Source: CAD feature listing. Evaluate the final solid. Frame: model axes, mm. Face numbers are marked on the shaded views. A direction names the side the tool comes from. Coordinates: 2 decimals unless noted, no trailing zeros. Write each loop counter-clockwise with the first axis right and the second up, starting at its lowest first coordinate (ties: lowest second). Pieces come first, ordered by that corner, then holes. Notation, with made-up numbers: M 10,68.25 L 31,68.25 A9 ccw 31,78.25 Z; hole C 11,43 d3. An arc over 180 degrees is marked long. One line per item, written item: value. Start each with the question number.
Item 1: Pin query (flat end, axial travel): P1, Ø8, axis at y = 16, z = 6, coming from the +X side; P2, Ø10, axis at x = 4, y = 18, coming from the +Z side; P3, Ø2.5, axis at y = 2, z = 0, coming from the +X side. Return the tip coordinate at first contact, or that it passes through.
Item 2: Set-up query: the marked faces 1 and 2. Return all of +Z, -Z, +X, -X, +Y, -Y with unobstructed straight access to the full face (end or side cutting, diameter ignored); none if empty.
Item 3: Cut plane A-A, the plane z = 0. Output: boundary loops of the cut face in (x, y), then the cut area to 3 significant figures.
Item 4: Cut plane C-C, the plane y = 4.5. Output: boundary loops of the cut face in (x, z).
Item 5: Cut plane B-B, the plane y = 16.25. Output: boundary loops of the cut face in (x, z).
Item 6: Mould query, pull axis X, two halves, no side actions, for the marked faces 3, 4 and 5. Classes: released by +X, released by -X, zero draft, split by the parting line, or undercut.
Item 7: Ray query, L1, parallel to Y at x = -4, z = -2.5; L2, parallel to X at y = 9, z = 0; L3, parallel to X at y = 7.5, z = 0. Return the intervals inside material, ascending. Write a range as from..to.
```python
from build123d import *

# Parameters (mm, degrees)
CUT_EXTRUDE1_DEPTH = 3.0988


with BuildPart() as part:
    # Sketch1 → Revolve1 (revolve)
    with BuildSketch(Plane.XY):
        Polygon((12.7, 0), (2.3622, 0), (2.3622, 20.828), (5.5372, 20.828), align=None)
    revolve(axis=Axis((0, 0, 0), (0, 1, 0)))

    # Sketch2 → Cut-Extrude1 (cut)
    with BuildSketch(Plane.XZ):
        Polygon((0, 5.381943739), (-4.6609, 2.69097187), (-4.6609, -2.69097187), (0, -5.381943739), (4.6609, -2.69097187), (4.6609, 2.69097187), align=None)
    extrude(amount=-CUT_EXTRUDE1_DEPTH, mode=Mode.SUBTRACT)


solid = part.part
```
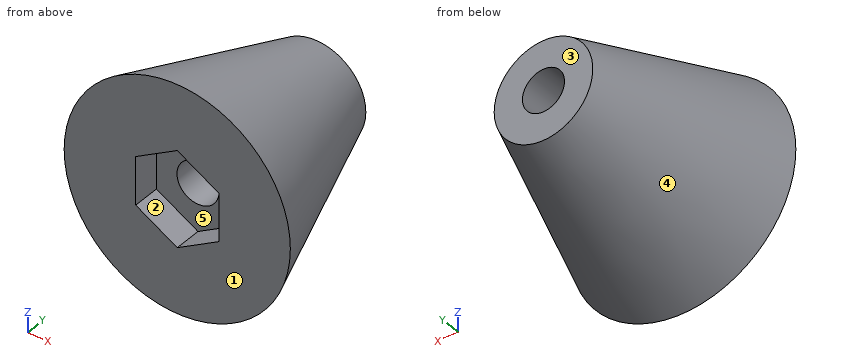
From the geometry:
1. P1: stops at x = 7.53
1. P2: stops at z = 7.86
1. P3: stops at x = 12.44
2. face 1: +Z, -Z, +X, -X, -Y
2. face 2: -Y
3. outline: M -12.7,0 L -4.66,0 L -4.66,3.1 L -2.36,3.1 L -2.36,20.83 L -5.54,20.83 Z; M 2.36,3.1 L 4.66,3.1 L 4.66,0 L 12.7,0 L 5.54,20.83 L 2.36,20.83 Z
3. area: 267 mm²
4. outline: C 0,0 d22.3; hole C 0,0 d4.72
5. outline: C 0,0 d14.22; hole C 0,0 d4.72
6. face 3: zero draft
6. face 4: split by the parting line
6. face 5: undercut
7. L1: y = 3.1..20.83
7. L2: x = -9.6..-2.36, 2.36..9.6
7. L3: x = -10.12..-2.36, 2.36..10.12
